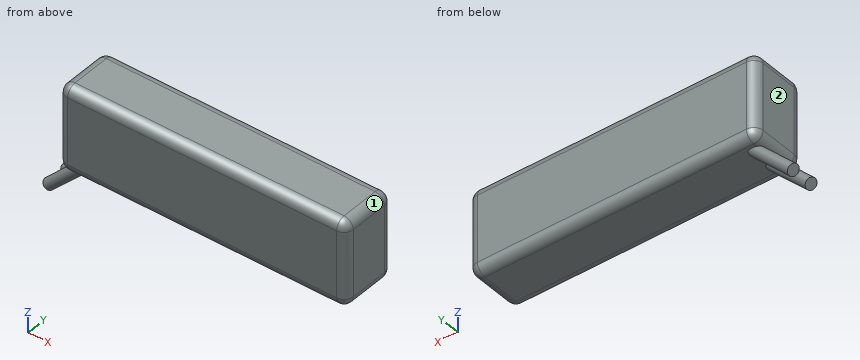
from build123d import *

# Parameters (mm, degrees)
SKETCH1_W           = 155
SKETCH1_H           = 46
BOSS_EXTRUDE1_DEPTH = 15.5
SKETCH4_R           = 3
BOSS_EXTRUDE2_DEPTH = 30
FILLET1_R           = 5


with BuildPart() as part:
    # Sketch1 → Boss-Extrude1 (new, symmetric)
    with BuildSketch(Plane(origin=(0, 0, 0), x_dir=(1, 0, 0), z_dir=(0, 1, 0))):
        Rectangle(SKETCH1_W, SKETCH1_H)
    extrude(amount=BOSS_EXTRUDE1_DEPTH, both=True)

    # Sketch4 → Boss-Extrude2 (add)
    with BuildSketch(Plane(origin=(-45.25, 0, -45.25), x_dir=(0.7071067811865509, 0, -0.7071067811865442), z_dir=(0.7071067811865442, 0, 0.7071067811865509))):
        with Locations((-33.537319575, 6)):
            Circle(SKETCH4_R)
        with Locations((-33.537319575, -6)):
            Circle(SKETCH4_R)
    extrude(amount=-BOSS_EXTRUDE2_DEPTH)

    # Fillet1
    # the kernel refuses this fillet: 5 mm, written as the material it takes off along each edge
    with BuildSketch(Plane(origin=(-72.5, 10.5, 18), x_dir=(0, 1, 0), z_dir=(-1, 0, 0))) as fillet1_piece_1_section:
        Polygon((0, 0), (FILLET1_R, 0), (FILLET1_R, -FILLET1_R), (0, -FILLET1_R), align=None)
    fillet1_piece_1 = extrude(amount=FILLET1_R, mode=Mode.PRIVATE)
    fillet1_piece_1 = fillet1_piece_1 - Plane(origin=(-72.5, 10.5, 18), x_dir=(0, -0.7071067811865475, -0.7071067811865475), z_dir=(-1, 0, 0)) * Sphere(FILLET1_R, mode=Mode.PRIVATE)
    add(fillet1_piece_1, mode=Mode.SUBTRACT)
    with BuildSketch(Plane(origin=(-72.5, 10.5, -18), x_dir=(-1, 0, 0), z_dir=(0, 0, -1))) as fillet1_piece_2_section:
        Polygon((0, 0), (FILLET1_R, 0), (FILLET1_R, FILLET1_R), (0, FILLET1_R), align=None)
    fillet1_piece_2 = extrude(amount=FILLET1_R, mode=Mode.PRIVATE)
    fillet1_piece_2 = fillet1_piece_2 - Plane(origin=(-72.5, 10.5, -18), x_dir=(0.7071067811865475, -0.7071067811865475, 0), z_dir=(0, 0, -1)) * Sphere(FILLET1_R, mode=Mode.PRIVATE)
    add(fillet1_piece_2, mode=Mode.SUBTRACT)
    with BuildSketch(Plane(origin=(72.5, 10.5, 18), x_dir=(0, 1, 0), z_dir=(0, 0, 1))) as fillet1_piece_3_section:
        Polygon((0, 0), (FILLET1_R, 0), (FILLET1_R, -FILLET1_R), (0, -FILLET1_R), align=None)
    fillet1_piece_3 = extrude(amount=FILLET1_R, mode=Mode.PRIVATE)
    fillet1_piece_3 = fillet1_piece_3 - Plane(origin=(72.5, 10.5, 18), x_dir=(-0.7071067811865475, -0.7071067811865475, 0), z_dir=(0, 0, 1)) * Sphere(FILLET1_R, mode=Mode.PRIVATE)
    add(fillet1_piece_3, mode=Mode.SUBTRACT)
    with BuildSketch(Plane(origin=(72.5, 10.5, -18), x_dir=(0, 1, 0), z_dir=(0, 0, -1))) as fillet1_piece_4_section:
        Polygon((0, 0), (FILLET1_R, 0), (FILLET1_R, FILLET1_R), (0, FILLET1_R), align=None)
    fillet1_piece_4 = extrude(amount=FILLET1_R, mode=Mode.PRIVATE)
    fillet1_piece_4 = fillet1_piece_4 - Plane(origin=(72.5, 10.5, -18), x_dir=(-0.7071067811865475, -0.7071067811865475, 0), z_dir=(0, 0, -1)) * Sphere(FILLET1_R, mode=Mode.PRIVATE)
    add(fillet1_piece_4, mode=Mode.SUBTRACT)
    with BuildSketch(Plane(origin=(72.5, -10.5, 18), x_dir=(0, -1, 0), z_dir=(0, 0, 1))) as fillet1_piece_5_section:
        Polygon((0, 0), (FILLET1_R, 0), (FILLET1_R, FILLET1_R), (0, FILLET1_R), align=None)
    fillet1_piece_5 = extrude(amount=FILLET1_R, mode=Mode.PRIVATE)
    fillet1_piece_5 = fillet1_piece_5 - Plane(origin=(72.5, -10.5, 18), x_dir=(-0.7071067811865475, 0.7071067811865475, 0), z_dir=(0, 0, 1)) * Sphere(FILLET1_R, mode=Mode.PRIVATE)
    add(fillet1_piece_5, mode=Mode.SUBTRACT)
    with BuildSketch(Plane(origin=(-72.5, -10.5, 18), x_dir=(0, -1, 0), z_dir=(0, 0, 1))) as fillet1_piece_6_section:
        Polygon((0, 0), (FILLET1_R, 0), (FILLET1_R, -FILLET1_R), (0, -FILLET1_R), align=None)
    fillet1_piece_6 = extrude(amount=FILLET1_R, mode=Mode.PRIVATE)
    fillet1_piece_6 = fillet1_piece_6 - Plane(origin=(-72.5, -10.5, 18), x_dir=(0.7071067811865475, 0.7071067811865475, 0), z_dir=(0, 0, 1)) * Sphere(FILLET1_R, mode=Mode.PRIVATE)
    add(fillet1_piece_6, mode=Mode.SUBTRACT)
    with BuildSketch(Plane(origin=(-72.5, -10.5, -18), x_dir=(-1, 0, 0), z_dir=(0, 0, -1))) as fillet1_piece_7_section:
        Polygon((0, 0), (FILLET1_R, 0), (FILLET1_R, -FILLET1_R), (0, -FILLET1_R), align=None)
    fillet1_piece_7 = extrude(amount=FILLET1_R, mode=Mode.PRIVATE)
    fillet1_piece_7 = fillet1_piece_7 - Plane(origin=(-72.5, -10.5, -18), x_dir=(0.7071067811865475, 0.7071067811865475, 0), z_dir=(0, 0, -1)) * Sphere(FILLET1_R, mode=Mode.PRIVATE)
    add(fillet1_piece_7, mode=Mode.SUBTRACT)
    with BuildSketch(Plane(origin=(72.5, -10.5, -18), x_dir=(0, -1, 0), z_dir=(0, 0, -1))) as fillet1_piece_8_section:
        Polygon((0, 0), (FILLET1_R, 0), (FILLET1_R, -FILLET1_R), (0, -FILLET1_R), align=None)
    fillet1_piece_8 = extrude(amount=FILLET1_R, mode=Mode.PRIVATE)
    fillet1_piece_8 = fillet1_piece_8 - Plane(origin=(72.5, -10.5, -18), x_dir=(-0.7071067811865475, 0.7071067811865475, 0), z_dir=(0, 0, -1)) * Sphere(FILLET1_R, mode=Mode.PRIVATE)
    add(fillet1_piece_8, mode=Mode.SUBTRACT)
    with BuildSketch(Plane(origin=(-77.5, 15.5, 18), x_dir=(0, -1, 0), z_dir=(0, 0, -1)), Plane(origin=(77.5, -15.5, -18), x_dir=(-1, 0, 0), z_dir=(0, 0, 1))) as fillet1_piece_9:
        with BuildLine():
            CenterArc((FILLET1_R, -FILLET1_R), FILLET1_R, 90, 90)
            Line((0, -FILLET1_R), (0, 0))
            Line((0, 0), (FILLET1_R, 0))
        make_face()
    extrude(amount=36, mode=Mode.SUBTRACT)
    with BuildSketch(Plane(origin=(72.5, 15.5, 23), x_dir=(0, 0, -1), z_dir=(-1, 0, 0)), Plane(origin=(-72.5, -15.5, -23), x_dir=(0, 1, 0), z_dir=(1, 0, 0))) as fillet1_piece_10:
        with BuildLine():
            CenterArc((FILLET1_R, FILLET1_R), FILLET1_R, 180, 90)
            Line((0, FILLET1_R), (0, 0))
            Line((0, 0), (FILLET1_R, 0))
        make_face()
    extrude(amount=145, mode=Mode.SUBTRACT)
    with BuildSketch(Plane(origin=(77.5, 15.5, -18), x_dir=(-1, 0, 0), z_dir=(0, 0, 1)), Plane(origin=(-77.5, -15.5, 18), x_dir=(0, 1, 0), z_dir=(0, 0, -1))) as fillet1_piece_11:
        with BuildLine():
            CenterArc((FILLET1_R, FILLET1_R), FILLET1_R, 180, 90)
            Line((0, FILLET1_R), (0, 0))
            Line((0, 0), (FILLET1_R, 0))
        make_face()
    extrude(amount=36, mode=Mode.SUBTRACT)
    with BuildSketch(Plane(origin=(72.5, -15.5, 23), x_dir=(0, 0, -1), z_dir=(-1, 0, 0)), Plane(origin=(-72.5, 15.5, -23), x_dir=(0, -1, 0), z_dir=(1, 0, 0))) as fillet1_piece_12:
        with BuildLine():
            CenterArc((FILLET1_R, -FILLET1_R), FILLET1_R, 90, 90)
            Line((0, -FILLET1_R), (0, 0))
            Line((0, 0), (FILLET1_R, 0))
        make_face()
    extrude(amount=145, mode=Mode.SUBTRACT)
    with BuildSketch(Plane(origin=(77.5, 10.5, 23), x_dir=(0, 0, -1), z_dir=(0, -1, 0)), Plane(origin=(-77.5, -10.5, 23), x_dir=(0, 0, -1), z_dir=(0, 1, 0)), Plane(origin=(77.5, 10.5, -23), x_dir=(-1, 0, 0), z_dir=(0, -1, 0))) as fillet1_piece_13:
        with BuildLine():
            CenterArc((FILLET1_R, -FILLET1_R), FILLET1_R, 90, 90)
            Line((0, -FILLET1_R), (0, 0))
            Line((0, 0), (FILLET1_R, 0))
        make_face()
    extrude(amount=21, mode=Mode.SUBTRACT)
    with BuildSketch(Plane(origin=(-77.5, -10.5, -23), x_dir=(1, 0, 0), z_dir=(0, 1, 0))) as fillet1_piece_14_section:
        with BuildLine():
            CenterArc((FILLET1_R, -FILLET1_R), FILLET1_R, 90, 90)
            Line((0, -FILLET1_R), (0, 0))
            Line((0, 0), (FILLET1_R, 0))
        make_face()
    fillet1_piece_14 = extrude(amount=21, mode=Mode.PRIVATE)
    fillet1_piece_14 = fillet1_piece_14 - Plane(origin=(-72.851968895, -6, -25.423036706), x_dir=(0.7071067811865509, 0, -0.7071067811865442), z_dir=(0.7071067811865442, 0, 0.7071067811865509)) * Cylinder(3, 62, mode=Mode.PRIVATE)
    fillet1_piece_14 = fillet1_piece_14 - Plane(origin=(-72.851968895, 6, -25.423036706), x_dir=(0.7071067811865509, 0, -0.7071067811865442), z_dir=(0.7071067811865442, 0, 0.7071067811865509)) * Cylinder(3, 62, mode=Mode.PRIVATE)
    add(fillet1_piece_14, mode=Mode.SUBTRACT)


solid = part.part
Here's how the part is built. I have some questions about the finished solid (model axes, mm). Face numbers are marked on the shaded views. A direction names the side the tool comes from. Coordinates: 2 decimals unless noted, no trailing zeros. Order: outer loops, then holes, each group sorted by start corner. A loop starts at its lowest first (then second) coordinate and runs counter-clockwise, first axis right, second up.
Item 1: For the marked faces 1 and 2, which set-ups out of +Z, -Z, +X, -X, +Y, -Y let a thin tool reach every point of the face, with its end or its side?
Result sheet:
face 1: +Z, +X, +Y, -Y
face 2: +Z, -X, +Y, -Y
Item 2: If we section it at B-B on z = -1.5: List the corners of the cut face in (x, y) for me, plus the area to 3 significant figures.
Result sheet:
outline: (-77.5, -10.5) arc R5 ccw to (-72.5, -15.5) - (72.5, -15.5) arc R5 ccw to (77.5, -10.5) - (77.5, 10.5) arc R5 ccw to (72.5, 15.5) - (-72.5, 15.5) arc R5 ccw to (-77.5, 10.5) - close
area: 4,780 mm2
Item 3: I need wall thicknesses on line 1 (X direction, y = -10, z = 3.5); line 2 (Z direction, x = -40, y = 6); line 3 (Y direction, x = -73, z = -17). Which ranges of each line are inside material? Lowest first, please.
Result sheet:
line 1: x = -77.5 to 77.5
line 2: z = -23 to 23
line 3: y = -15.47 to 15.47
Item 4: If we section it at A-A on x = 66: List the corners of the cut face in (y, z) for me.
Result sheet:
outline: (-15.5, -18) arc R5 ccw to (-10.5, -23) - (10.5, -23) arc R5 ccw to (15.5, -18) - (15.5, 18) arc R5 ccw to (10.5, 23) - (-10.5, 23) arc R5 ccw to (-15.5, 18) - close
Item 5: For P1, Ø6.5, axis at y = 4.5, z = -6, coming from the -X side; P2, Ø4, axis at x = -6, z = -21, coming from the -Y side; P3, Ø1.5, axis at x = 41.5, y = -10, coming from the -Z side, each with a flat end and sliding along its axis, tell me the tip position at first contact or that it passes through.
Result sheet:
P1: stops at x = -77.5
P2: stops at y = -15.4
P3: stops at z = -23
